Answer from the drawing. Dimensions are ordinates in mm from the lowest x, y and z of the part. Round coordinates to 2 decimals unless told otherwise and drop trailing zeros. Write each loop counter-clockwise with the first axis right and the second up, starting at its lowest first coordinate (ties: lowest second). Pieces come first, ordered by that corner, then holes. Notation, with made-up numbers: (35, -27) - (71, -27) arc R25 cw to (71, -2) - close; hole circle Ø6 at (21, 73). An arc over 180 degrees is marked (long way). Answer in a Markdown table with one row per item.
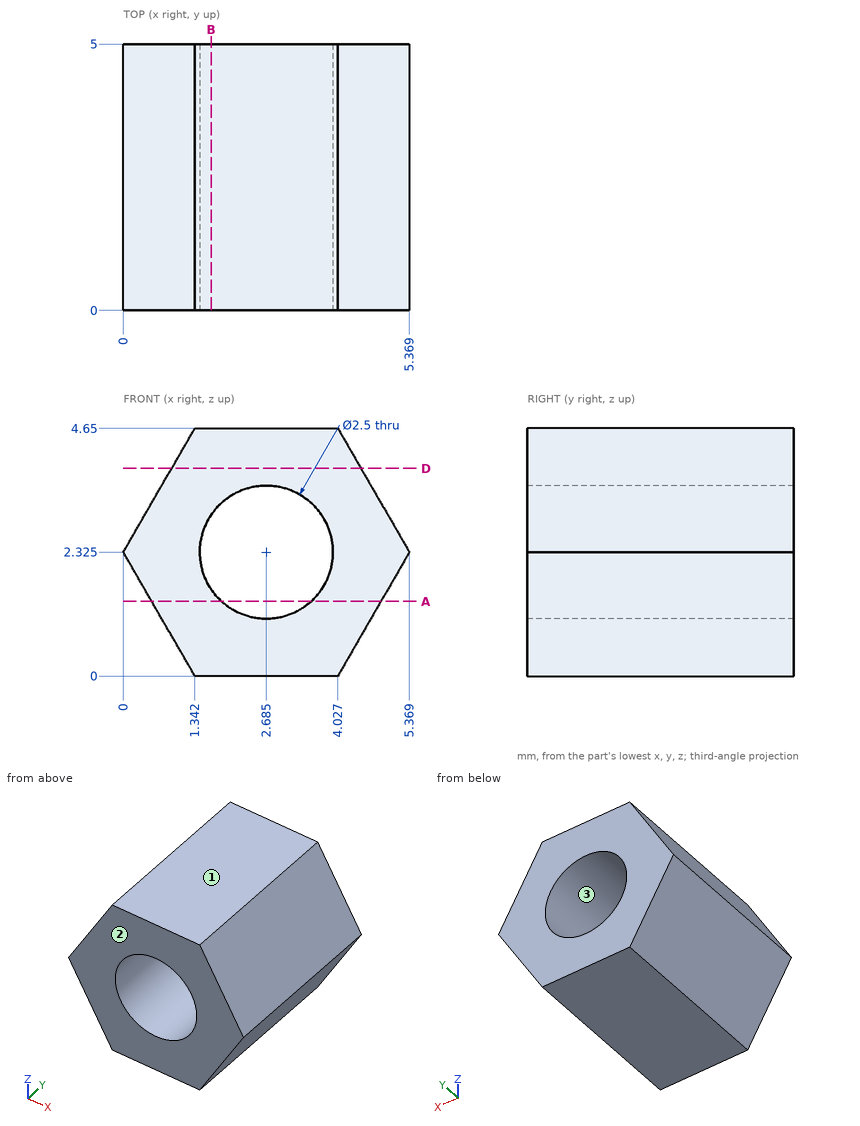
(1) Flat-ended cylindrical pins translate along their axes: pin 1 (2 mm diameter, centred on x = 2.68, z = 2.33, fed in from -Y); pin 2 (1 mm diameter, centred on y = 3.5, z = 3.5, fed in from -X); pin 3 (2 mm diameter, centred on y = 2, z = 3.5, fed in from -X); pin 4 (1 mm diameter, centred on y = 3.5, z = 1, fed in from +X). Find the tip coordinate at first contact, or state that the pin passes through.
Checked values:
| item | result |
|---|---|
| pin 1 | passes through |
| pin 2 | stops at x = 0.39 |
| pin 3 | stops at x = 0.1 |
| pin 4 | stops at x = 4.89 |
(2) Find the intervals of material crossed by line 1 (Z direction, x = 2.1, y = 2.4); line 2 (X direction, y = 4.65, z = 2.15); line 3 (X direction, y = 4.65, z = 2.9) (1 decimal), in increasing order.
Checked values:
| item | result |
|---|---|
| line 1 | z = 0 to 1.22, 3.43 to 4.65 |
| line 2 | x = 0.1 to 1.45, 3.92 to 5.27 |
| line 3 | x = 0.3 to 1.6, 3.8 to 5 |
(3) Section A-A (z = 1.4) is taken. Give the vertices of the cut face in (x, y) (1 decimal), and give its area (3 significant figures).
Checked values:
| item | result |
|---|---|
| outline | (0.5, 0) - (1.8, 0) - (1.8, 5) - (0.5, 5) - close; (3.5, 0) - (4.8, 0) - (4.8, 5) - (3.5, 5) - close |
| area | 13.1 mm2 |
(4) Section D-D (z = 3.9) is taken. Give the vertices of the cut face in (x, y).
Checked values:
| item | result |
|---|---|
| outline | (0.91, 0) - (4.46, 0) - (4.46, 5) - (0.91, 5) - close |
(5) Section B-B (x = 1.65) is taken. Give the vertices of the cut face in (y, z).
Checked values:
| item | result |
|---|---|
| outline | (0, 0) - (5, 0) - (5, 1.62) - (0, 1.62) - close; (0, 3.03) - (5, 3.03) - (5, 4.65) - (0, 4.65) - close |
(6) For a pull along Z with two mould halves and no side action, classify the marked faces 1, 2 and 3 as pulls with the +Z half, pulls with the -Z half, needs draft (parallel to the pull), parting line crosses it, or undercut.
Checked values:
| item | result |
|---|---|
| face 1 | pulls with the +Z half |
| face 2 | needs draft |
| face 3 | undercut |
